Autodesk Inventor part; units mm, degrees
ref_plane "YZ Plane" through (0, 0, 0) normal (1, 0, 0) x (0, 1, 0)
ref_plane "XZ Plane" through (0, 0, 0) normal (0, 1, 0) x (-1, 0, 0)
ref_plane "XY Plane" through (0, 0, 0) normal (0, 0, 1) x (1, 0, 0)
sketch "Sketch1" plane through (0, 0, 0) normal (0, 1, 0) x (-1, 0, 0)
  line L0 (25.527, 20.828) -> (-25.527, 20.828)
  line L1 (-25.527, 20.828) -> (-25.527, -20.828)
  line L2 (-25.527, -20.828) -> (25.527, -20.828)
  line L3 (25.527, -20.828) -> (25.527, 20.828)
  circle A0 centre (18.9992, 13.3858) radius 1.9837
  circle A1 centre (18.9992, -13.3858) radius 1.9837
  circle A2 centre (-18.9992, -13.3858) radius 1.9837
  circle A3 centre (-18.9992, 13.3858) radius 1.9837
  circle A4 centre (18.9992, 13.3858) radius 3.048 construction
  point P0 (0, 0)
  point P1 (25.527, 0)
  point P2 (0, -20.828)
  dimension "d0" = 3.9675
  dimension "d1" = 41.656
  dimension "d2" = 51.054
  dimension "d3" = 6.096
  dimension "d4" = 7.4422
  dimension "d5" = 6.5278
  dimension "d6" = 7.4422
  dimension "d7" = 6.5278
sketch "Sketch10" plane through (0, 0, 0) normal (0, 0, 1) x (1, 0, 0)
  line L0 (-25.527, 0) -> (25.527, 0)
  line L1 (25.527, 0) -> (25.527, 7.6416)
  line L2 (-25.527, 0) -> (-25.527, 3.175)
  line L3 (-25.527, 3.175) -> (25.527, 7.6416)
  point P0 (0, 0)
  dimension "d61" = 5
  dimension "d62" = 3.175
extrude "Extrusion8" add sketch "Sketch10" along normal mid plane 41.656
sketch "Sketch11" plane through (-25.527, 0, 20.828) normal (0, -1, 0) x (1, 0, 0)
  line L0 (46.1137, -7.4422) -> (42.9387, -7.4422) construction
  line L1 (46.1137, -4.9149) -> (42.9387, -4.9149)
  line L2 (42.9387, -9.9695) -> (46.1137, -9.9695)
  arc A0 (46.1137, -9.9695) -> (46.1137, -4.9149) centre (46.1137, -7.4422) ccw
  arc A1 (42.9387, -4.9149) -> (42.9387, -9.9695) centre (42.9387, -7.4422) ccw
  line L3 (46.1137, -34.2138) -> (42.9387, -34.2138) construction
  line L4 (51.054, -41.656) -> (51.054, 0)
  line L5 (46.1137, -36.7411) -> (42.9387, -36.7411)
  line L6 (42.9387, -31.6865) -> (46.1137, -31.6865)
  arc A2 (46.1137, -36.7411) -> (46.1137, -31.6865) centre (46.1137, -34.2138) ccw
  arc A3 (42.9387, -31.6865) -> (42.9387, -36.7411) centre (42.9387, -34.2138) ccw
  line L7 (8.1153, -34.2138) -> (4.9403, -34.2138) construction
  line L8 (8.1153, -36.7411) -> (4.9403, -36.7411)
  line L9 (4.9403, -31.6865) -> (8.1153, -31.6865)
  arc A4 (8.1153, -36.7411) -> (8.1153, -31.6865) centre (8.1153, -34.2138) ccw
  arc A5 (4.9403, -31.6865) -> (4.9403, -36.7411) centre (4.9403, -34.2138) ccw
  line L10 (8.1153, -7.4422) -> (4.9403, -7.4422) construction
  line L11 (8.1153, -9.9695) -> (4.9403, -9.9695)
  line L12 (4.9403, -4.9149) -> (8.1153, -4.9149)
  arc A6 (8.1153, -9.9695) -> (8.1153, -4.9149) centre (8.1153, -7.4422) ccw
  arc A7 (4.9403, -4.9149) -> (4.9403, -9.9695) centre (4.9403, -7.4422) ccw
  point P0 (25.527, -20.828)
  point P1 (44.5262, -7.4422)
  point P2 (44.5262, -34.2138)
  point P3 (6.5278, -34.2138)
  point P4 (6.5278, -7.4422)
  point P5 (44.5262, -7.4422)
  point P6 (44.5262, -34.2138)
  point P7 (6.5278, -34.2138)
  point P8 (6.5278, -7.4422)
  point P9 (44.5262, -9.9695)
  point P10 (6.5278, -36.7411)
  dimension "d65" = 3.175
  dimension "d66" = 2.5273
extrude "Extrusion9" cut sketch "Sketch11" against normal blind 41.656
sketch "Sketch13" plane through (25.527, 0, 20.828) normal (1, 0, 0) x (0, 0, -1)
  line L0 (41.656, 7.6416) -> (0, 7.6416)
  line L1 (0, 0) -> (0, 7.6416)
  line L2 (41.656, 0) -> (0, 0)
  line L3 (41.656, 7.6416) -> (41.656, 0)
  line L4 (25.4999, 2.032) -> (16.1561, 2.032)
  spline S0 degree 2 poles (20.8859, 3.1075) (20.8859, 2.8579) (20.7161, 2.436) (20.5488, 2.2841) knots 0 0 0 1 2 2 2
  spline S1 degree 2 poles (20.5488, 2.2841) (20.3816, 2.1323) (19.9236, 1.9651) (19.5891, 1.9651) knots 0 0 0 1 2 2 2
  spline S2 degree 2 poles (19.5891, 1.9651) (19.2341, 1.9677) (18.7246, 2.0835) (18.5574, 2.1581) knots 0 0 0 1 2 2 2
  line L5 (18.5574, 2.1581) -> (18.5574, 2.8502)
  line L6 (18.5574, 2.8502) -> (18.6294, 2.8502)
  spline S3 degree 2 poles (18.6294, 2.8502) (18.6912, 2.8167) (18.8404, 2.7293) (18.9613, 2.683) knots 0 0 0 1 2 2 2
  spline S4 degree 2 poles (18.9613, 2.683) (19.0745, 2.6392) (19.3087, 2.58) (19.4502, 2.58) knots 0 0 0 1 2 2 2
  spline S5 degree 2 poles (19.4502, 2.58) (19.5737, 2.58) (19.8619, 2.6418) (19.9493, 2.7241) knots 0 0 0 1 2 2 2
  spline S6 degree 2 poles (19.9493, 2.7241) (20.0137, 2.7884) (20.0857, 2.9454) (20.0857, 3.0766) knots 0 0 0 1 2 2 2
  spline S7 degree 2 poles (20.0857, 3.0766) (20.0857, 3.1898) (19.9931, 3.3493) (19.9185, 3.3982) knots 0 0 0 1 2 2 2
  spline S8 degree 2 poles (19.9185, 3.3982) (19.8104, 3.4703) (19.5017, 3.5114) (19.391, 3.5114) knots 0 0 0 1 2 2 2
  spline S9 degree 2 poles (19.391, 3.5114) (19.2161, 3.5114) (18.8841, 3.4548) (18.7632, 3.424) knots 0 0 0 1 2 2 2
  line L7 (18.7632, 3.424) -> (18.6938, 3.424)
  line L8 (18.6938, 3.424) -> (18.6938, 5.207)
  line L9 (18.6938, 5.207) -> (20.7984, 5.207)
  line L10 (20.7984, 5.207) -> (20.7984, 4.6075)
  line L11 (20.7984, 4.6075) -> (19.4476, 4.6075)
  line L12 (19.4476, 4.6075) -> (19.4476, 4.0801)
  spline S10 degree 2 poles (19.4476, 4.0801) (19.5119, 4.0852) (19.6895, 4.0903) (19.7384, 4.0903) knots 0 0 0 1 2 2 2
  spline S11 degree 2 poles (19.7384, 4.0903) (19.9674, 4.0903) (20.3533, 3.9977) (20.5051, 3.9025) knots 0 0 0 1 2 2 2
  spline S12 degree 2 poles (20.5051, 3.9025) (20.6852, 3.7842) (20.8859, 3.3905) (20.8859, 3.1075) knots 0 0 0 1 2 2 2
  spline S13 degree 2 poles (23.0832, 4.4145) (23.0832, 4.0518) (22.5789, 3.5552) (22.2187, 3.5552) knots 0 0 0 1 2 2 2
  spline S14 degree 2 poles (22.2187, 3.5552) (21.8559, 3.5552) (21.3516, 4.0518) (21.3516, 4.4145) knots 0 0 0 1 2 2 2
  spline S15 degree 2 poles (21.3516, 4.4145) (21.3516, 4.7773) (21.8559, 5.2739) (22.2187, 5.2739) knots 0 0 0 1 2 2 2
  spline S16 degree 2 poles (22.2187, 5.2739) (22.5815, 5.2739) (23.0832, 4.7773) (23.0832, 4.4145) knots 0 0 0 1 2 2 2
  spline S17 degree 2 poles (22.6175, 4.4145) (22.6175, 4.5818) (22.3885, 4.8211) (22.2187, 4.8211) knots 0 0 0 1 2 2 2
  spline S18 degree 2 poles (22.2187, 4.8211) (22.0489, 4.8211) (21.8173, 4.5844) (21.8173, 4.4145) knots 0 0 0 1 2 2 2
  spline S19 degree 2 poles (21.8173, 4.4145) (21.8173, 4.2396) (22.0514, 4.008) (22.2187, 4.008) knots 0 0 0 1 2 2 2
  spline S20 degree 2 poles (22.2187, 4.008) (22.3885, 4.008) (22.6175, 4.2447) (22.6175, 4.4145) knots 0 0 0 1 2 2 2
  point P0 (20.828, 0)
  point P1 (20.828, 0)
  point P2 (20.828, 2.032)
  dimension "d69" = 2.032
extrude "Extrusion10" cut sketch "Sketch13" against normal blind 0.381 contours S1 S2 L4 | L4 S2 L5 L6 S3 S4 S5 S6 S7 S8 S9 L7 L8 L9 L10 L11 L12 S10 S11 S12 S0 S1 | S13 S14 S15 S16
equation "\"d6\" = d4"
equation "\"d7\" = d5"
equation "\"d23\" = d22"
equation "\"d25\" = 0.5 * d24"
properties part number "shim 5 Deg"
Part model, mm, in its own coordinate system. A direction names the side the tool comes from. Round coordinates to 2 decimals unless told otherwise and drop trailing zeros. Loops run counter-clockwise (first coordinate to the right, second up) from the corner with the lowest first, then second, coordinate; pieces in that order, holes last.
Item 1: Cut at B-B, the plane x = -18. Give the cut face in (y, z).
Item 2: Cut at A-A, the plane z = -12.5. Give the cut face in (x, y) (3 decimals).
Item 3: Drill centre lines: line 1 (X direction, y = 1, z = -14.5); line 2 (X direction, y = 1.25, z = -11.5); line 3 (Z direction, x = 22, y = 2.75). Where is each one in solid material? Low to high.
Item 4: Mould opens along X. For faces 3 (the face through (-25.527, 2, 0)), 4 (the face through (25.527, 4, 0)), 5 (the face through (23.113, 3.664, 13.33)) say: +X half, -X half, draft (parallel to the pull), parting line (faces both ways), or undercut.
Item 5: Cut at D-D, the plane z = 5. Give the cut face in (x, y) (3 decimals).
Item 6: 3-axis set-ups, long thin cutter, end or side, ignore diameter. For faces 1 (the face through (25.146, 4, -1)), 2 (the face through (19, 4, 15.913)): which of +Z, -Z, +X, -X, +Y, -Y reach the whole face in a straight line?
Item 7: Drop flat-ended pins along their axis: P1, Ø2, axis at x = -18, z = -16, coming from the +Y side; P2, Ø5, axis at x = -9.5, z = 8.5, coming from the +Y side; P3, Ø8, axis at x = 12, z = -14, coming from the +Y side. Give the stop position or say it passes through.
Item 8: Cut at C-C, the plane y = 6. Give the cut face in (x, z), then the cut area to 3 significant figures.
A:
1. outline: (0, -20.83) - (3.83, -20.83) - (3.83, -15.91) - (0, -15.91) - close; (0, -10.86) - (3.83, -10.86) - (3.83, 10.86) - (0, 10.86) - close; (0, 15.91) - (3.83, 15.91) - (3.83, 20.83) - (0, 20.83) - close
2. outline: (-25.527, 0) - (-22.954, 0) - (-22.954, 3.4) - (-25.527, 3.175) - close; (-15.045, 0) - (15.045, 0) - (15.045, 6.725) - (-15.045, 4.092) - close; (22.954, 0) - (25.527, 0) - (25.527, 7.642) - (22.954, 7.416) - close
3. line 1: x = -25.53 to -22.86, -15.14 to 15.14, 22.86 to 25.53
3. line 2: x = -25.53 to -22.27, -15.73 to 15.73, 22.27 to 25.53
3. line 3: z = -20.83 to -15.48, -11.29 to 11.29, 15.48 to 20.83
4. face 3: -X half
4. face 4: +X half
4. face 5: undercut
5. outline: (-25.527, 0) - (25.527, 0) - (25.527, 7.642) - (-25.527, 3.175) - close
6. face 1: +X
6. face 2: +Y, -Y
7. P1: stops at y = 3.92
7. P2: stops at y = 4.8
7. P3: stops at y = 6.79
8. outline: (6.76, -20.83) - (25.53, -20.83) - (25.53, 20.83) - (6.76, 20.83) - close; hole (17.41, -15.91) - (20.59, -15.91) arc R2.53 ccw to (20.59, -10.86) - (17.41, -10.86) arc R2.53 ccw to start; hole (17.41, 10.86) - (20.59, 10.86) arc R2.53 ccw to (20.59, 15.91) - (17.41, 15.91) arc R2.53 ccw to start
8. area: 709 mm2
